Autodesk Inventor part; units mm, degrees
ref_plane "YZ Plane" through (0, 0, 0) normal (1, 0, 0) x (0, 1, 0)
ref_plane "XZ Plane" through (0, 0, 0) normal (0, 1, 0) x (-1, 0, 0)
ref_plane "XY Plane" through (0, 0, 0) normal (0, 0, 1) x (1, 0, 0)
sketch "Skizze1" plane through (0, 0, 0) normal (1, 0, 0) x (0, 1, 0)
  line L0 (0, 0) -> (-10, 0) construction
  circle A0 centre (0, 0) radius 1.1
  circle A1 centre (-10, 0) radius 1.1
  arc A2 (-10, 2.5) -> (-10, -2.5) centre (-10, 0) ccw
  line L1 (-10, -2.5) -> (3.8, -2.5)
  line L2 (-10, 2.5) -> (1.8, 2.5)
  arc A3 (3.8, 0.5) -> (1.8, 2.5) centre (1.8, 0.5) ccw
  line L3 (3.8, 0.5) -> (3.8, -2.5)
  dimension "d0" = 10
  dimension "d1" = 2.2
  dimension "d2" = 2.2
  dimension "d3" = 2.5
  dimension "d8" = 2
  dimension "d9" = 3.8
extrude "Extrusion1" add sketch "Skizze1" along normal mid plane 4
chamfer "Fase1" distance 0.5 angle 45 10 edges at (2, 3.2142, 1.9142) (2, -4.1, 2.5) (2, -12.5, 0) (2, -3.1, -2.5) (2, 3.8, -1) (-2, 3.2142, 1.9142) (-2, -4.1, 2.5) (-2, -12.5, 0) (-2, -3.1, -2.5) (-2, 3.8, -1)
sketch "Skizze4" plane through (-1.5, -10, 2.5) normal (0, 0, 1) x (1, 0, 0)
  line L0 (1.5, 17.06) -> (1.5, -5.76) construction
  line L1 (0, 0) -> (3, 0) construction
  line L2 (0.75, 0.4) -> (2.25, 0.4)
  line L3 (2.25, 0.4) -> (2.25, 0)
  line L4 (2.25, 0) -> (0.75, 0)
  line L5 (0.75, 0) -> (0.75, 0.4)
  line L6 (0.75, 0.4) -> (2.25, 0) construction
  line L7 (2.25, 0.4) -> (0.75, 0) construction
  point P0 (1.5, 10)
  point P1 (1.5, 0.2)
  point P2 (1.5, 0)
  dimension "d23" = 0.4
  dimension "d24" = 1.5
extrude "Extrusion3" cut sketch "Skizze4" against normal blind 0.2
pattern_linear "Rechteckige Anordnung1" count 4 spacing 1 along (0, 1, 0) of "Extrusion3"
equation "\"d2\" = d1"
properties part number "Chipanschlag T2"
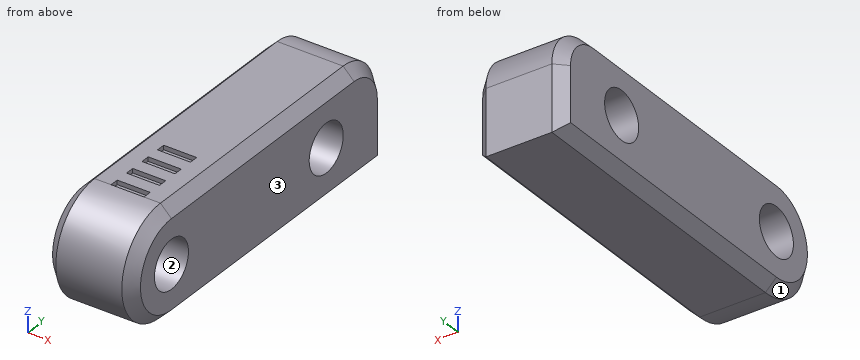
CAD build for the part. Positions are in the model's coordinates, mm. Face numbers are marked on the shaded views. Round coordinates to 2 decimals unless told otherwise and drop trailing zeros. Order: outer loops, then holes, each group sorted by start corner. A loop starts at its lowest first (then second) coordinate and runs counter-clockwise, first axis right, second up.
Item 1: Saw through at C-C on x = -0.55. Write the cut outline in (y, z), then the cut area to 3 significant figures.
Item 2: Pin check, flat tip, straight feed: pin 1 (2 mm diameter, centred on x = -1, z = 1.5, fed in from -Y). Stop position of the tip, or through.
Item 3: Saw through at A-A on z = 0. Write the cut outline in (x, y).
Item 4: Saw through at D-D on y = -7.75. Write the cut outline in (x, z).
Item 5: Mould opens along Y. For the marked faces 1, 2 and 3 say: pulls with the +Y half, pulls with the -Y half, needs draft (parallel to the pull), parting line crosses it, or undercut.
Item 6: Probe line 1 along Y through (x, z) = (1.8, 0.4); line 2 along Y through (x, z) = (1.85, -0.3); line 3 along Z through (x, y) = (0.65, -10.75). List the from-to ranges inside material, lowest first.
Item 7: Saw through at B-B on y = 0. Write the cut outline in (x, z).
Reported:
1. outline: (-10, -2.5) - (3.8, -2.5) - (3.8, 0.5) arc R2 ccw to (1.8, 2.5) - (-6.6, 2.5) - (-6.6, 2.3) - (-7, 2.3) - (-7, 2.5) - (-7.6, 2.5) - (-7.6, 2.3) - (-8, 2.3) - (-8, 2.5) - (-8.6, 2.5) - (-8.6, 2.3) - (-9, 2.3) - (-9, 2.5) - (-9.6, 2.5) - (-9.6, 2.3) - (-10, 2.3) - (-10, 2.5) arc R2.5 ccw to start; hole circle Ø2.2 at (-10, 0); hole circle Ø2.2 at (0, 0)
1. area: 70.0 mm2
2. pin 1: stops at y = -12.45
3. outline: (-2, -12) - (-1.5, -12.5) - (1.5, -12.5) - (2, -12) - (2, -11.1) - (-2, -11.1) - close; (-2, -8.9) - (2, -8.9) - (2, -1.1) - (-2, -1.1) - close; (-2, 1.1) - (2, 1.1) - (2, 3.3) - (1.5, 3.8) - (-1.5, 3.8) - (-2, 3.3) - close
4. outline: (-2, -2) - (-1.5, -2.5) - (1.5, -2.5) - (2, -2) - (2, 2) - (1.5, 2.5) - (0.75, 2.5) - (0.75, 2.3) - (-0.75, 2.3) - (-0.75, 2.5) - (-1.5, 2.5) - (-2, 2) - close
5. face 1: pulls with the -Y half
5. face 2: undercut
5. face 3: needs draft
6. line 1: y = -12.16 to -11.02, -8.98 to -1.02, 1.02 to 3.5
6. line 2: y = -12.13 to -11.06, -8.94 to -1.06, 1.06 to 3.45
6. line 3: z = -2.38 to -0.8, 0.8 to 2.38
7. outline: (-2, -2) - (-1.5, -2.5) - (1.5, -2.5) - (2, -2) - (2, -1.1) - (-2, -1.1) - close; (-2, 1.1) - (2, 1.1) - (2, 2) - (1.5, 2.5) - (-1.5, 2.5) - (-2, 2) - close
